Autodesk Inventor part; units mm, degrees
ref_plane "Work Plane1" through (0, 0, 4) normal (0, 0, 1) x (1, 0, 0)
ref_plane "YZ Plane" through (0, 0, 0) normal (1, 0, 0) x (0, 1, 0)
ref_plane "XZ Plane" through (0, 0, 0) normal (0, 1, 0) x (-1, 0, 0)
sketch "Sketch1" plane through (0, 0, 0) normal (0, 0, 1) x (1, 0, 0)
  line L0 (0, 0) -> (50, 0)
  line L1 (50, 0) -> (50, -25)
  line L2 (50, -25) -> (0, -25)
  line L3 (0, -25) -> (0, 0)
  line L4 (50, 0) -> (60, 0)
  line L5 (60, -25) -> (50, -25)
  line L6 (0, -25) -> (-10, -25)
  line L7 (-10, 0) -> (0, 0)
  circle A0 centre (55, -12.5) radius 1.15
  circle A1 centre (-5, -12.5) radius 1.15
  line L8 (-10, 0) -> (-10, -25)
  line L9 (60, 0) -> (60, -25)
  point P0 (60, -12.5)
  point P1 (-10, -12.5)
  dimension "d0" = 50
  dimension "d1" = 25
  dimension "d19" = 10
  dimension "d20" = 10
  dimension "d21" = 2.3
  dimension "d22" = 2.3
  dimension "d37" = 12.5
  dimension "d38" = 12.5
  dimension "d39" = 12.5
  dimension "d40" = 5
  dimension "d41" = 5
  dimension "d42" = 12.5
  dimension "d43" = 12.5
extrude "Extrusion1" add sketch "Sketch1" along normal blind 2
sketch "Sketch4" plane through (0, 0, 2) normal (0, 0, 1) x (1, 0, 0)
  line L0 (2.15, -22.85) -> (47.85, -22.85)
  line L1 (47.85, -22.85) -> (47.85, -2.15)
  line L2 (47.85, -2.15) -> (2.15, -2.15)
  line L3 (2.15, -2.15) -> (2.15, -22.85)
  line L4 (60, -25) -> (60, 0)
  point P0 (0, 0)
  point P1 (2.15, -12.5)
  point P2 (50, -25)
  dimension "d25" = 20.7
  dimension "d26" = 2.15
  dimension "d27" = 45.7
  dimension "d44" = 12.15
ref_plane "Work Plane1" through (0, 0, 4) normal (0, 0, 1) x (1, 0, 0)
sketch "Sketch5" plane through (0, 0, 4) normal (0, 0, 1) x (1, 0, 0)
  line L0 (31, -25) -> (19, -25)
  line L1 (19, -25) -> (19, -17)
  line L2 (19, -17) -> (31, -17)
  line L3 (31, -17) -> (31, -25)
  line L4 (-10, -25) -> (60, -25)
  line L5 (-10, 0) -> (-10, -25)
  point P0 (0, 0)
  dimension "d32" = 12
  dimension "d33" = 8
  dimension "d50" = 29
fillet "Fillet1" radius 4 4 edges at (-10, 0, 1) (60, 0, 1) (-10, -25, 1) (60, -25, 1)
extrude "Extrusion6" add sketch "Sketch4" along normal blind 2
extrude "Extrusion7" cut sketch "Sketch5" against normal through all
properties part number "UltrasonicSensorMountTest_backplate"
Read the model definition and answer for the solid it produces. Units are mm, in the model's axes. A direction names the side the tool comes from. Coordinates: 2 decimals unless noted, no trailing zeros. Loops run counter-clockwise (first coordinate to the right, second up) from the corner with the lowest first, then second, coordinate; pieces in that order, holes last.
(1) The mould has two halves that part along X. Classify faces 1 (the face through (31, -21, 2)), 2 (the face through (25, -12, 4)), 3 (the face through (58.859, -1.203, 1.014)): released by +X, released by -X, zero draft, split by the parting line, or undercut.
Solution:
face 1: undercut
face 2: zero draft
face 3: released by +X
(2) The part is cut by section D-D (x = 3.5). Determine the outline of the cut face in (y, z).
Solution:
outline: (-25, 0) - (0, 0) - (0, 2) - (-2.15, 2) - (-2.15, 4) - (-22.85, 4) - (-22.85, 2) - (-25, 2) - close
(3) The part is cut by section C-C (z = 3.05). Determine the outline of the cut face in (x, y), and give its area (3 significant figures).
Solution:
outline: (2.15, -22.85) - (19, -22.85) - (19, -17) - (31, -17) - (31, -22.85) - (47.85, -22.85) - (47.85, -2.15) - (2.15, -2.15) - close
area: 876 mm2
(4) The part is cut by section A-A (y = -12.5). Determine the outline of the cut face in (x, z), and give its area (3 significant figures).
Solution:
outline: (-10, 0) - (-6.15, 0) - (-6.15, 2) - (-10, 2) - close; (-3.85, 0) - (53.85, 0) - (53.85, 2) - (47.85, 2) - (47.85, 4) - (2.15, 4) - (2.15, 2) - (-3.85, 2) - close; (56.15, 0) - (60, 0) - (60, 2) - (56.15, 2) - close
area: 222 mm2
(5) Flat-ended cylindrical pins translate along their axes: pin 1 Ø1.4 at (x, y) = (55, -12.5) entering from -Z; pin 2 Ø0.6 at (x, z) = (32.5, 2.5) entering from +Y; pin 3 Ø1.2 at (y, z) = (-20, 3) entering from +X; pin 4 Ø2.5 at (x, y) = (-5, -12.5) entering from +Z. Find the tip coordinate at first contact, or state that the pin passes through.
Solution:
pin 1: passes through
pin 2: stops at y = -2.15
pin 3: stops at x = 47.85
pin 4: stops at z = 2
(6) Consider line 1 along Y through (x, z) = (55, 1.4); line 2 along Y through (x, z) = (38.5, 2.25); line 3 along Y through (x, z) = (25.5, 2.35). Determine where each line is inside the solid, lowest interval first.
Solution:
line 1: y = -25 to -13.65, -11.35 to 0
line 2: y = -22.85 to -2.15
line 3: y = -17 to -2.15
(7) A tool of negligible diameter and unlimited length cuts with its end or side. For faces 4 (the face through (2.15, -12, 3)), 5 (the face through (25, -2.15, 3)), 6 (the face through (39, -22.85, 3)), from which of +Z, -Z, +X, -X, +Y, -Y can it reach the whole face along a straight path? Write none if from no direction.
Solution:
face 4: +Z, -X, +Y, -Y
face 5: +Z, +X, -X, +Y
face 6: +Z, +X, -X, -Y
(8) The part is cut by section B-B (x = -5). Determine the outline of the cut face in (y, z), and give its area (3 significant figures).
Solution:
outline: (-25, 0) - (-13.65, 0) - (-13.65, 2) - (-25, 2) - close; (-11.35, 0) - (0, 0) - (0, 2) - (-11.35, 2) - close
area: 45.4 mm2
